from build123d import *

# Parameters (mm, degrees)
EXTRUDE_T_DEPTH        = 15
SKETCH_937_W           = 118.457051
SKETCH_937_H           = 10
EXTRUDE_1_DEPTH        = 15
FILLET_1172_R          = 5
FILLET_1670_R          = 10
FILLET_1882_R          = 10
SKETCH_2094_R          = 1.5
CUT_EXTRUDE_2102_DEPTH = 244.711622867


with BuildPart() as part:
    # Эскиз t → t (new body)
    with BuildSketch(Plane(origin=(0, 0, 0), x_dir=(1, 0, 0), z_dir=(0, 1, 0))):
        with BuildLine():
            Line((0, 153.846153846), (40.13974359, 153.846153846))
            Line((40.13974359, 153.846153846), (40.13974359, 200))
            Line((40.13974359, 200), (81.686217949, 200))
            Line((81.686217949, 200), (81.686217949, 153.846153846))
            Line((81.686217949, 153.846153846), (138.457051282, 153.846153846))
            Line((138.457051282, 153.846153846), (138.457051282, 117.548076923))
            Line((138.457051282, 117.548076923), (81.686217949, 117.548076923))
            Line((81.686217949, 117.548076923), (81.686217949, 52.243589744))
            add(Edge.make_bspline(
                [(81.686217949, 52.243589744), (81.655267201, 49.982948441), (82.085389497, 46.690532241), (83.817672815, 42.793259528), (85.603921155, 40.439849904), (87.847865612, 38.561179508), (91.543310131, 36.686733749), (94.758311571, 36.350436228), (96.910576923, 36.298076923)],
                knots=[0, 0, 0, 0, 0.27148881, 0.391200884, 0.507818538, 0.622673608, 0.739445184, 1, 1, 1, 1], degree=3))
            Line((96.910576923, 36.298076923), (135.692628205, 36.298076923))
            Line((135.692628205, 36.298076923), (135.692628205, 0))
            Line((135.692628205, 0), (92.743910256, 0))
            add(Edge.make_bspline(
                [(92.743910256, 0), (88.849192705, 0.050339472), (83.116455127, 0.365762726), (75.810535171, 1.898538288), (70.797203285, 3.478754574), (66.08408468, 5.454229708), (61.749524849, 7.981859361), (57.691359691, 10.855934374), (54.053352032, 14.254057303), (50.767538722, 18.006446438), (47.908525609, 22.119844392), (45.483732962, 26.56295255), (43.519863299, 31.361705258), (42.002327108, 36.504881897), (40.54984301, 43.989384334), (40.084701759, 49.821816441), (40.13974359, 53.806089744)],
                knots=[0, 0, 0, 0, 0.137098935, 0.200908089, 0.261934675, 0.321669044, 0.380133534, 0.437984068, 0.496125333, 0.554687761, 0.613033376, 0.671858669, 0.73227727, 0.794962552, 0.860057524, 1, 1, 1, 1], degree=3))
            Line((40.13974359, 53.806089744), (40.13974359, 117.548076923))
            Line((40.13974359, 117.548076923), (0, 117.548076923))
            Line((0, 117.548076923), (0, 153.846153846))
        make_face()
    extrude(amount=EXTRUDE_T_DEPTH)

    # Sketch 937 → Вытянуть-Тонкостенный1 (add)
    with BuildSketch(Plane(origin=(0, 0, 0), x_dir=(1, 0, 0), z_dir=(0, 1, 0))):
        with BuildLine():
            Line((55.913237, 190), (55.913237, 49.511337503))
            ThreePointArc((55.913237, 49.511337503), (66.563507798, 23.799309298), (92.275536003, 13.1490385))
            Line((92.275536003, 13.1490385), (125.697051, 13.1490385))
            Line((125.697051, 13.1490385), (125.697051, 23.1490385))
            Line((125.697051, 23.1490385), (92.275536003, 23.1490385))
            ThreePointArc((92.275536003, 23.1490385), (73.63457561, 30.87037711), (65.913237, 49.511337503))
            Line((65.913237, 49.511337503), (65.913237, 190))
            Line((65.913237, 190), (55.913237, 190))
        make_face()
        with Locations((69.2285255, 135.6990385)):
            Rectangle(SKETCH_937_W, SKETCH_937_H)
    extrude(amount=-EXTRUDE_1_DEPTH)

    # Fillet 1172
    fillet_1172_edges = [part.edges().sort_by_distance(p)[0] for p in [
        (128.457051, -7.5, -140.6990385),
        (128.457051, -7.5, -130.6990385),
        (125.697051, -7.5, -23.1490385),
        (125.697051, -7.5, -13.1490385),
        (10, -7.5, -130.6990385),
        (10, -7.5, -140.6990385),
        (55.913237, -7.5, -190),
        (65.913237, -7.5, -190),
    ]]
    fillet(fillet_1172_edges, radius=FILLET_1172_R - 0.0001)  # a hair under: the kernel refuses the full size

    # Fillet 1670
    fillet_1670_edges = [part.edges().sort_by_distance(p)[0] for p in [
        (55.913237, -7.5, -140.6990385),
        (65.913237, -7.5, -130.6990385),
        (65.913237, -7.5, -140.6990385),
        (55.913237, -7.5, -130.6990385),
    ]]
    fillet(fillet_1670_edges, radius=FILLET_1670_R)

    # Fillet 1882
    fillet_1882_edges = [part.edges().sort_by_distance(p)[0] for p in [
        (40.13974359, 7.5, -153.846153846),
        (81.686217949, 7.5, -153.846153846),
        (81.686217949, 7.5, -117.548076923),
        (40.13974359, 7.5, -117.548076923),
    ]]
    fillet(fillet_1882_edges, radius=FILLET_1882_R)

    # Sketch 2094 → Cut-Extrude 2102 (cut, through all)
    with BuildSketch(Plane(origin=(0, 0, 0), x_dir=(1, 0, 0), z_dir=(0, 1, 0))):
        with Locations(Location((60.913237, 135.699039, 0), (0, 0, 270))):
            Circle(SKETCH_2094_R)
        with Locations(Location((120.697051, 18.149039, 0), (0, 0, 270))):
            Circle(SKETCH_2094_R)
        with Locations(Location((123.457051, 135.699039, 0), (0, 0, 270))):
            Circle(SKETCH_2094_R)
    extrude(amount=-CUT_EXTRUDE_2102_DEPTH, mode=Mode.SUBTRACT)


solid = part.part
The model under review builds one solid part; all positions refer to its coordinate system, in mm. A direction names the side the tool comes from. Give positions to 0.01 mm unless a question says otherwise; leave off trailing zeros. Loops run counter-clockwise (first coordinate to the right, second up) from the corner with the lowest first, then second, coordinate; pieces in that order, holes last. Notation, with made-up numbers: (66, 34) -> (78, 34) arc R28 cw to (78, 68) -> close; hole circle Ø9 at (68.5, 88.25). An arc over 180 degrees is marked (long way). Write each question's results on one line, items separated by ' | '.
1) Take a section at B-B, the plane z = -65. Give the boundary of the cut face in (x, y), plus the area to 3 significant figures.
Conclusion:
outline: (40.14, 0) -> (55.91, 0) -> (55.91, -15) -> (65.91, -15) -> (65.91, 0) -> (81.69, 0) -> (81.69, 15) -> (40.14, 15) -> close | area: 773 mm^2
2) Draft analysis for pull direction Z (two halves, no side actions). For faces 5 (the face through (70, 0, -101)), 6 (the face through (64.487, -7.605, -188.496)), 7 (the face through (115, 7, 0)), state which applies: pulls with the +Z half, pulls with the -Z half, needs draft (parallel to the pull), parting line crosses it, or undercut.
Conclusion:
face 5: undercut | face 6: pulls with the -Z half | face 7: pulls with the +Z half
3) Tool access review of faces 1 (the face through (107, -7, -23.149)), 2 (the face through (52.906, -7.605, -127.847)), 3 (the face through (106, -7, -13.149)), 4 (the face through (53.062, -7.605, -143.706)): name each direction out of +Z, -Z, +X, -X, +Y, -Y from which nothing blocks a thin tool from reaching the whole face with its end or side.
Conclusion:
face 1: +X, -Y | face 2: +Z, -X, -Y | face 3: +Z, +X, -X, -Y | face 4: -Z, -X, -Y
4) Take a section at A-A, the plane x = 112. Give the boundary of the cut face in (y, z).
Conclusion:
outline: (-15, -140.7) -> (0, -140.7) -> (0, -153.85) -> (15, -153.85) -> (15, -117.55) -> (0, -117.55) -> (0, -130.7) -> (-15, -130.7) -> close; (-15, -23.15) -> (0, -23.15) -> (0, -36.3) -> (15, -36.3) -> (15, 0) -> (0, 0) -> (0, -13.15) -> (-15, -13.15) -> close
5) Take a section at D-D, the plane z = -112. Give the boundary of the cut face in (x, y), plus the area to 3 significant figures.
Conclusion:
outline: (39.09, 0) -> (55.91, 0) -> (55.91, -15) -> (65.91, -15) -> (65.91, 0) -> (82.73, 0) -> (82.73, 15) -> (39.09, 15) -> close | area: 805 mm^2
6) For line 1 along Z through (x, y) = (128.5, 14); line 2 along Y through (x, z) = (45.5, -57); line 3 along X through (y, z) = (3, -83.5), list the stretches that pass through material, from the lowest coordinate up. Write a range as from..to.
Conclusion:
line 1: z = -153.85..-117.55, -36.3..0 | line 2: y = 0..15 | line 3: x = 40.14..81.69
7) Take a section at C-C, the plane y = -5. Count the separate pieces of the cut face and the enclosed holes in it, plus the area to 3 significant figures.
Conclusion:
separate pieces: 1 | enclosed holes: 3 | area: 3,340 mm^2
8) Insertion check: pin 1 Ø16.5 at (y, z) = (7, -183) entering from +X; pin 2 Ø7.5 at (y, z) = (9, -178.5) entering from -X; pin 3 Ø1.5 at (x, y) = (61.5, 5.5) entering from +Z. Each pin has a flat end and moves straight along its axis. Give the tip position at first contact, or say it passes through.
Conclusion:
pin 1: stops at x = 81.69 | pin 2: stops at x = 40.14 | pin 3: stops at z = -7.75
